from build123d import *

# Parameters (mm, degrees)
BASES_W            = 23
BASES_H            = 44
BASE_DEPTH         = 3.3
BASE_F_R           = 0.5
POCKETS_W          = 21.4
POCKETS_H          = 42.4
CUT_EXTRUDE3_DEPTH = 26.686767021


with BuildPart() as part:
    # BaseS → BASE (new, symmetric)
    with BuildSketch(Plane(origin=(0, 0, 0), x_dir=(1, 0, 0), z_dir=(0, 1, 0))):
        Rectangle(BASES_W, BASES_H)
    extrude(amount=BASE_DEPTH, both=True)

    # BASE F
    base_f_edges = [part.edges().sort_by_distance(p)[0] for p in [
        (11.5, 0, 22),
        (-11.5, 0, 22),
        (-11.5, 0, -22),
        (11.5, 0, -22),
    ]]
    fillet(base_f_edges, radius=BASE_F_R)

    # PocketS → Cut-Extrude3 (cut, through all)
    with BuildSketch(Plane(origin=(0, 3.3, 0), x_dir=(1, 0, 0), z_dir=(0, 1, 0))):
        Rectangle(POCKETS_W, POCKETS_H)
    extrude(amount=-CUT_EXTRUDE3_DEPTH, mode=Mode.SUBTRACT)


solid = part.part
Could you check a few things on this model? Use its own coordinates, in mm. A direction names the side the tool comes from. Round coordinates to 2 decimals unless told otherwise and drop trailing zeros. Order: outer loops, then holes, each group sorted by start corner. A loop starts at its lowest first (then second) coordinate and runs counter-clockwise, first axis right, second up. Notation, with made-up numbers: M 70.25,52.5 L 112.25,52.5 A18 cw 112.25,85.5 Z; hole C -6,79 d4. An arc over 180 degrees is marked long. One line per item, written item: value.
(1) Imagine slicing it at A-A (z = 14.5). Write out the boundary of the cut face in (x, y).
Ans:
outline: M -11.5,-3.3 L -10.7,-3.3 L -10.7,3.3 L -11.5,3.3 Z; M 10.7,-3.3 L 11.5,-3.3 L 11.5,3.3 L 10.7,3.3 Z
(2) Imagine slicing it at B-B (x = 6.25). Write out the boundary of the cut face in (y, z).
Ans:
outline: M -3.3,-22 L 3.3,-22 L 3.3,-21.2 L -3.3,-21.2 Z; M -3.3,21.2 L 3.3,21.2 L 3.3,22 L -3.3,22 Z
(3) If we mould it in two halves opening along X, with no side actions, what happens to faces 3 (the flat face through (10.7, 0, 0)), 4 (the flat face through (11, 3.3, -7)), 5 (the flat face through (-11.5, 0, 0))? For each: released by +X, released by -X, zero draft, split by the parting line, or undercut.
Ans:
face 3: undercut
face 4: zero draft
face 5: released by -X
(4) Imagine slicing it at C-C (y = 0.75). Write out the boundary of the cut face in (x, z), and give its area (3 significant figures).
Ans:
outline: M -11.5,-21.5 A0.5 ccw -11,-22 L 11,-22 A0.5 ccw 11.5,-21.5 L 11.5,21.5 A0.5 ccw 11,22 L -11,22 A0.5 ccw -11.5,21.5 Z; hole M -10.7,-21.2 L 10.7,-21.2 L 10.7,21.2 L -10.7,21.2 Z
area: 104 mm^2
(5) I need wall thicknesses on line 1 along Z through (x, y) = (2.25, 0.5); line 2 along X through (y, z) = (0.25, -15.5). Which ranges of each line are inside material? Lowest first, please. Write a range as from..to.
Ans:
line 1: z = -22..-21.2, 21.2..22
line 2: x = -11.5..-10.7, 10.7..11.5
(6) Which directions (+Z, -Z, +X, -X, +Y, -Y) give clear straight access to the entire face, cutting with the end or side of a thin tool? Please do faces 1 (the flat face through (0, 0, -21.2)), 2 (the flat face through (0, 0, 22)).
Ans:
face 1: +Y, -Y
face 2: +Z, +X, -X, +Y, -Y
